```python
from build123d import *

# Parameters (mm, degrees)
SKETCH_4_R          = 64
EXTRUDE_1_DEPTH     = 7
SKETCH_5_R          = 37.5
SKETCH_5_R_2        = 32.5
EXTRUDE_2_DEPTH     = 12
SKETCH_7_R          = 12.5
CUT_EXTRUDE_1_DEPTH = 92.301697684
FILLET_1_R          = 2
SKETCH_10_R         = 13.5
EXTRUDE_3_DEPTH     = 30
SKETCH_11_R         = 7.5
CUT_EXTRUDE_2_DEPTH = 96.351979528
FILLET_2_R          = 2


with BuildPart() as part:
    # 草图4 → 凸台-拉伸1 (new body)
    with BuildSketch(Plane(origin=(0, 0, 0), x_dir=(1, 0, 0), z_dir=(0, 1, 0))):
        with Locations(Location((0, 0, 0), (0, 0, 270))):
            Circle(SKETCH_4_R)
    extrude(amount=EXTRUDE_1_DEPTH)

    # 草图5 → 凸台-拉伸2 (add)
    with BuildSketch(Plane(origin=(0, 7, 0), x_dir=(1, 0, 0), z_dir=(0, 1, 0))):
        with Locations(Location((0, 0, 0), (0, 0, 270))):
            Circle(SKETCH_5_R)
        with Locations(Location((0, 0, 0), (0, 0, 270))):
            Circle(SKETCH_5_R_2, mode=Mode.SUBTRACT)
    extrude(amount=EXTRUDE_2_DEPTH)

    # 草图7 → 切除-拉伸1 (cut, through all)
    with BuildSketch(Plane(origin=(0, 7, 0), x_dir=(1, 0, 0), z_dir=(0, 1, 0))):
        with Locations(Location((0, 0, 0), (0, 0, 270))):
            Circle(SKETCH_7_R)
    extrude(amount=-CUT_EXTRUDE_1_DEPTH, mode=Mode.SUBTRACT)

    # 圆角1
    fillet_1_edges = [part.edges().sort_by_distance(p)[0] for p in [
        (0, 19, -32.5),
        (0, 19, -37.5),
    ]]
    fillet(fillet_1_edges, radius=FILLET_1_R)

    # 草图10 → 凸台-拉伸3 (add)
    with BuildSketch(Plane(origin=(0, 0, 0), x_dir=(1, 0, 0), z_dir=(0, 1, 0))):
        with Locations(Location((0, 35, 0), (0, 0, 359.939369671))):
            Circle(SKETCH_10_R)
    extrude(amount=EXTRUDE_3_DEPTH)

    # 草图11 → 切除-拉伸2 (cut, through all)
    with BuildSketch(Plane(origin=(0, 30, 0), x_dir=(1, 0, 0), z_dir=(0, 1, 0))):
        with Locations(Location((0, 35, 0), (0, 0, 270))):
            Circle(SKETCH_11_R)
    extrude(amount=-CUT_EXTRUDE_2_DEPTH, mode=Mode.SUBTRACT)

    # 圆角2
    fillet_2_edges = [part.edges().sort_by_distance(p)[0] for p in [
        (-13.499992441, 30, -35.014285682),
        (0, 30, -42.5),
    ]]
    fillet(fillet_2_edges, radius=FILLET_2_R)


solid = part.part
```
Part model, mm, in its own coordinate system. A direction names the side the tool comes from. Round coordinates to 2 decimals unless told otherwise and drop trailing zeros. Loops run counter-clockwise (first coordinate to the right, second up) from the corner with the lowest first, then second, coordinate; pieces in that order, holes last. Notation, with made-up numbers: (-33, 1) -> (2, 1) arc R29 cw to (2, 25) -> close; hole circle Ø6 at (55.5, -11.75). An arc over 180 degrees is marked (long way). Use a Markdown table: item, result.
1) Pull direction Z, two halves, no side cores. Call faces 3 (the cylindrical face through (-1.46, 11.93, 37.47)), 4 (the flat face through (0, 7, 15)), 5 (the flat face through (-28, 7, 28)): pulls with the +Z half, pulls with the -Z half, needs draft (parallel to the pull), parting line crosses it, or undercut.
The answers:
| item | result |
|---|---|
| face 3 | parting line crosses it |
| face 4 | undercut |
| face 5 | needs draft |
2) Tool access for faces 1 (the cylindrical face through (-1.743, 17.353, -48.387)), 2 (the cylindrical face through (0.33, 14.196, -42.493)): list every direction of +Z, -Z, +X, -X, +Y, -Y with a clear straight run to the whole face (end or side of a thin tool).
The answers:
| item | result |
|---|---|
| face 1 | +Y |
| face 2 | +Y, -Y |
3) Probe line 1 (X direction, y = 4.5, z = 0); line 2 (X direction, y = 8, z = -35); line 3 (Y direction, x = -54, z = 22.5). List the from-to ranges inside material, lowest first. Write a range as [from, to].
The answers:
| item | result |
|---|---|
| line 1 | x = [-64, -12.5], [12.5, 64] |
| line 2 | x = [-13.5, -7.5], [7.5, 13.5] |
| line 3 | y = [0, 7] |
4) Cut at B-B, the plane z = 0. List the corners of the cut face in (x, y).
The answers:
| item | result |
|---|---|
| outline | (-64, 0) -> (-12.5, 0) -> (-12.5, 7) -> (-32.5, 7) -> (-32.5, 17) arc R2 ccw to (-34.5, 19) -> (-35.5, 19) arc R2 ccw to (-37.5, 17) -> (-37.5, 7) -> (-64, 7) -> close; (12.5, 0) -> (64, 0) -> (64, 7) -> (37.5, 7) -> (37.5, 17) arc R2 ccw to (35.5, 19) -> (34.5, 19) arc R2 ccw to (32.5, 17) -> (32.5, 7) -> (12.5, 7) -> close |
5) Cut at A-A, the plane x = 0. List the corners of the cut face in (y, z), and give its area (3 significant figures).
The answers:
| item | result |
|---|---|
| outline | (0, -64) -> (7, -64) -> (7, -48.5) -> (28, -48.5) arc R2 ccw to (30, -46.5) -> (30, -44.5) arc R2 ccw to (28, -42.5) -> (0, -42.5) -> close; (0, -27.5) -> (28, -27.5) arc R2 ccw to (30, -25.5) -> (30, -23.5) arc R2 ccw to (28, -21.5) -> (7, -21.5) -> (7, -12.5) -> (0, -12.5) -> close; (0, 12.5) -> (7, 12.5) -> (7, 32.5) -> (17, 32.5) arc R2 ccw to (19, 34.5) -> (19, 35.5) arc R2 ccw to (17, 37.5) -> (7, 37.5) -> (7, 64) -> (0, 64) -> close |
| area | 947 mm2 |
6) Cut at D-D, the plane z = 53.5. List the corners of the cut face in (x, y).
The answers:
| item | result |
|---|---|
| outline | (-35.12, 0) -> (35.12, 0) -> (35.12, 7) -> (-35.12, 7) -> close |
7) Drop flat-ended pins along their axis: pin 1 Ø8 at (x, y) = (-38, 14) entering from +Z; pin 2 Ø2 at (x, y) = (0, 19.5) entering from -Z; pin 3 Ø8 at (x, y) = (-27, 9.5) entering from +Z; pin 4 Ø10 at (x, z) = (-42, 42.5) entering from -Y. Give the stop position or say it passes through.
The answers:
| item | result |
|---|---|
| pin 1 | stops at z = 15.82 |
| pin 2 | stops at z = -48.5 |
| pin 3 | stops at z = 59.38 |
| pin 4 | stops at y = 0 |
8) Cut at C-C, the plane y = 21.5. List the corners of the cut face in (x, z).
The answers:
| item | result |
|---|---|
| outline | circle Ø27 at (0, -35); hole circle Ø15 at (0, -35) |
